```python
from build123d import *

# Parameters (mm, degrees)
SKETCH_1_R               = 1.5
SKETCH_1_R_2             = 9
SKETCH_1_R_3             = 2
EXTRUDE_1_DEPTH          = 2
CUT_EXTRUDE_1_DEPTH      = 100.85333965
CUT_EXTRUDE_1_DEPTH_BACK = 100.85333965
SKETCH_2_R               = 1.5
CUT_EXTRUDE_2_DEPTH      = 100.85333965
CUT_EXTRUDE_2_DEPTH_BACK = 100.85333965


with BuildPart() as part:
    # 草图1 → 凸台-拉伸1 (new body)
    with BuildSketch(Plane(origin=(0, 0, 0), x_dir=(1, 0, 0), z_dir=(0, 1, 0))):
        with BuildLine():
            Line((0, 47), (75.321800738, 47))
            ThreePointArc((75.321800738, 47), (76.607375957, 46.532088886), (77.291416244, 45.347296355))
            Line((77.291416244, 45.347296355), (88.047362067, -15.652703645))
            ThreePointArc((88.047362067, -15.652703645), (87.609835447, -17.285575219), (86.077746561, -18))
            Line((86.077746561, -18), (64.077746561, -18))
            ThreePointArc((64.077746561, -18), (48.289235397, -21.406433974), (35.309770387, -31.019673035))
            ThreePointArc((35.309770387, -31.019673035), (-42.818948099, -19.378794691), (0, 47))
        make_face()
        with Locations(Location((-16.264045876, 39.264880132, 0), (0, 0, 270))):
            Circle(SKETCH_1_R, mode=Mode.SUBTRACT)
        with Locations(Location((16.264045876, 39.264880132, 0), (0, 0, 270))):
            Circle(SKETCH_1_R, mode=Mode.SUBTRACT)
        with Locations(Location((39.264880132, -16.264045876, 0), (0, 0, 270))):
            Circle(SKETCH_1_R, mode=Mode.SUBTRACT)
        with Locations(Location((16.264045876, -39.264880132, 0), (0, 0, 270))):
            Circle(SKETCH_1_R, mode=Mode.SUBTRACT)
        with Locations(Location((-16.264045876, -39.264880132, 0), (0, 0, 270))):
            Circle(SKETCH_1_R, mode=Mode.SUBTRACT)
        with Locations(Location((-39.264880132, -16.264045876, 0), (0, 0, 270))):
            Circle(SKETCH_1_R, mode=Mode.SUBTRACT)
        with Locations(Location((-39.264880132, 16.264045876, 0), (0, 0, 270))):
            Circle(SKETCH_1_R, mode=Mode.SUBTRACT)
        with Locations(Location((0, 0, 0), (0, 0, 270))):
            Circle(SKETCH_1_R_2, mode=Mode.SUBTRACT)
        with Locations(Location((-6.783865663, 11.75, 0), (0, 0, 270))):
            Circle(SKETCH_1_R, mode=Mode.SUBTRACT)
        with Locations(Location((6.783865663, 11.75, 0), (0, 0, 270))):
            Circle(SKETCH_1_R, mode=Mode.SUBTRACT)
        with Locations(Location((13.567731326, 0, 0), (0, 0, 270))):
            Circle(SKETCH_1_R, mode=Mode.SUBTRACT)
        with Locations(Location((6.783865663, -11.75, 0), (0, 0, 270))):
            Circle(SKETCH_1_R, mode=Mode.SUBTRACT)
        with Locations(Location((-6.783865663, -11.75, 0), (0, 0, 270))):
            Circle(SKETCH_1_R, mode=Mode.SUBTRACT)
        with Locations(Location((-13.567731326, 0, 0), (0, 0, 270))):
            Circle(SKETCH_1_R, mode=Mode.SUBTRACT)
        with Locations(Location((0, 13.856406461, 0), (0, 0, 270))):
            Circle(SKETCH_1_R_3, mode=Mode.SUBTRACT)
        with Locations(Location((-12, -6.92820323, 0), (0, 0, 270))):
            Circle(SKETCH_1_R_3, mode=Mode.SUBTRACT)
        with Locations(Location((12, -6.92820323, 0), (0, 0, 270))):
            Circle(SKETCH_1_R_3, mode=Mode.SUBTRACT)
    extrude(amount=EXTRUDE_1_DEPTH)

    # 草图2 → 切除-拉伸1 (cut, two sides: drawn at the far end of the back side and taken through both)
    with BuildSketch(Plane(origin=(0, 2, 0), x_dir=(1, 0, 0), z_dir=(0, 1, 0)).offset(-CUT_EXTRUDE_1_DEPTH_BACK)):
        with Locations(Location((74.70156336, 37, 0), (0, 0, 270))):
            Circle(SKETCH_2_R)
        with Locations(Location((78.668920425, 14.5, 0), (0, 0, 270))):
            Circle(SKETCH_2_R)
        with Locations(Location((82.636277491, -8, 0), (0, 0, 270))):
            Circle(SKETCH_2_R)
        with Locations(Location((38.146205332, 37, 0), (0, 0, 270))):
            Circle(SKETCH_2_R)
        with Locations(Location((46.080919464, -8, 0), (0, 0, 270))):
            Circle(SKETCH_2_R)
        with Locations(Location((42.113562398, 14.5, 0), (0, 0, 270))):
            Circle(SKETCH_2_R)
        with BuildLine():
            Line((64.216309798, 27.359582102), (68.383866062, 3.72419603))
            ThreePointArc((68.383866062, 3.72419603), (63.51690861, -3.226539554), (56.566173025, 1.640417898))
            Line((56.566173025, 1.640417898), (52.398616761, 25.27580397))
            ThreePointArc((52.398616761, 25.27580397), (57.265574214, 32.226539554), (64.216309798, 27.359582102))
        make_face()
    extrude(amount=CUT_EXTRUDE_1_DEPTH + CUT_EXTRUDE_1_DEPTH_BACK, mode=Mode.SUBTRACT)

    # 草图3 → 切除-拉伸2 (cut, two sides: drawn at the far end of the back side and taken through both)
    with BuildSketch(Plane.XZ.offset(-CUT_EXTRUDE_2_DEPTH_BACK)):
        with BuildLine():
            ThreePointArc((7.550595775, -18.519948797), (12.17522858, -15.867066806), (15.934658856, -12.086630926))
            ThreePointArc((15.934658856, -12.086630926), (18.33030278, -10.583005244), (21.121590627, -11.039855496))
            Line((21.121590627, -11.039855496), (29.830018752, -16.067668818))
            ThreePointArc((29.830018752, -16.067668818), (31.73567133, -18.668128181), (31.104138605, -21.829625778))
            ThreePointArc((31.104138605, -21.829625778), (23.132934302, -30.147426931), (13.035455865, -35.694213682))
            ThreePointArc((13.035455865, -35.694213682), (9.818230989, -35.485971662), (7.799599311, -32.972204212))
            Line((7.799599311, -32.972204212), (5.197011625, -23.259214737))
            ThreePointArc((5.197011625, -23.259214737), (5.478166623, -20.44479617), (7.550595775, -18.519948797))
        make_face()
        with BuildLine():
            ThreePointArc((-12.263448247, -15.798982153), (-7.653668647, -18.47759065), (-2.5, -19.843134833))
            ThreePointArc((-2.5, -19.843134833), (0, -21.166010489), (1, -23.8117618))
            Line((1, -23.8117618), (1, -33.867388444))
            ThreePointArc((1, -33.867388444), (-0.29923758, -36.817961668), (-3.352941176, -37.851787084))
            ThreePointArc((-3.352941176, -37.851787084), (-14.54197043, -35.107422235), (-24.394367884, -29.13614277))
            ThreePointArc((-24.394367884, -29.13614277), (-25.822637443, -26.245823287), (-24.654966811, -23.240753248))
            Line((-24.654966811, -23.240753248), (-17.544565022, -16.130351459))
            ThreePointArc((-17.544565022, -16.130351459), (-14.966629547, -14.966629547), (-12.263448247, -15.798982153))
        make_face()
        with BuildLine():
            ThreePointArc((-19.814044022, 2.720966644), (-19.828897227, -2.610523844), (-18.434658856, -7.756503907))
            ThreePointArc((-18.434658856, -7.756503907), (-18.33030278, -10.583005244), (-20.121590627, -12.771906304))
            Line((-20.121590627, -12.771906304), (-28.830018752, -17.799719626))
            ThreePointArc((-28.830018752, -17.799719626), (-32.03490891, -18.149833488), (-34.457079782, -16.022161306))
            ThreePointArc((-34.457079782, -16.022161306), (-37.674904732, -4.959995304), (-37.429823749, 6.558070912))
            ThreePointArc((-37.429823749, 6.558070912), (-35.640868431, 9.240148374), (-32.454566122, 9.731450963))
            Line((-32.454566122, 9.731450963), (-22.741576647, 7.128863277))
            ThreePointArc((-22.741576647, 7.128863277), (-20.44479617, 5.478166623), (-19.814044022, 2.720966644))
        make_face()
        with BuildLine():
            ThreePointArc((-7.550595775, 18.519948797), (-12.17522858, 15.867066806), (-15.934658856, 12.086630926))
            ThreePointArc((-15.934658856, 12.086630926), (-18.33030278, 10.583005244), (-21.121590627, 11.039855496))
            Line((-21.121590627, 11.039855496), (-29.830018752, 16.067668818))
            ThreePointArc((-29.830018752, 16.067668818), (-31.73567133, 18.668128181), (-31.104138605, 21.829625778))
            ThreePointArc((-31.104138605, 21.829625778), (-23.132934302, 30.147426931), (-13.035455865, 35.694213682))
            ThreePointArc((-13.035455865, 35.694213682), (-9.818230989, 35.485971662), (-7.799599311, 32.972204212))
            Line((-7.799599311, 32.972204212), (-5.197011625, 23.259214737))
            ThreePointArc((-5.197011625, 23.259214737), (-5.478166623, 20.44479617), (-7.550595775, 18.519948797))
        make_face()
        with BuildLine():
            ThreePointArc((12.263448247, 15.798982153), (7.653668647, 18.47759065), (2.5, 19.843134833))
            ThreePointArc((2.5, 19.843134833), (0, 21.166010489), (-1, 23.8117618))
            Line((-1, 23.8117618), (-1, 33.867388444))
            ThreePointArc((-1, 33.867388444), (0.29923758, 36.817961668), (3.352941176, 37.851787084))
            ThreePointArc((3.352941176, 37.851787084), (14.54197043, 35.107422235), (24.394367884, 29.13614277))
            ThreePointArc((24.394367884, 29.13614277), (25.822637443, 26.245823287), (24.654966811, 23.240753248))
            Line((24.654966811, 23.240753248), (17.544565022, 16.130351459))
            ThreePointArc((17.544565022, 16.130351459), (14.966629547, 14.966629547), (12.263448247, 15.798982153))
        make_face()
        with BuildLine():
            ThreePointArc((19.814044022, -2.720966644), (19.828897227, 2.610523844), (18.434658856, 7.756503907))
            ThreePointArc((18.434658856, 7.756503907), (18.33030278, 10.583005244), (20.121590627, 12.771906304))
            Line((20.121590627, 12.771906304), (28.830018752, 17.799719626))
            ThreePointArc((28.830018752, 17.799719626), (32.03490891, 18.149833488), (34.457079782, 16.022161306))
            ThreePointArc((34.457079782, 16.022161306), (37.674904732, 4.959995304), (37.429823749, -6.558070912))
            ThreePointArc((37.429823749, -6.558070912), (35.640868431, -9.240148374), (32.454566122, -9.731450963))
            Line((32.454566122, -9.731450963), (22.741576647, -7.128863277))
            ThreePointArc((22.741576647, -7.128863277), (20.44479617, -5.478166623), (19.814044022, -2.720966644))
        make_face()
    extrude(amount=CUT_EXTRUDE_2_DEPTH + CUT_EXTRUDE_2_DEPTH_BACK, mode=Mode.SUBTRACT)


solid = part.part
```
Input: part model. Units: mm. Frame: model coordinates. Round coordinates to 2 decimals unless told otherwise and drop trailing zeros. Loops run counter-clockwise (first coordinate to the right, second up) from the corner with the lowest first, then second, coordinate; pieces in that order, holes last. Notation, with made-up numbers: M 39,58.25 L 61,58.25 A38 ccw 61,96.25 Z; hole C 3,-38.5 d3. An arc over 180 degrees is marked long. Answer in a Markdown table with one row per item. Add a question column.
1. Mould query, pull axis X, two halves, no side actions, for faces 1 (the face through (36, 0, -11)), 2 (the face through (12, 1, -16)). Classes: released by +X, released by -X, zero draft, split by the parting line, or undercut.
2. Ray query, probe 1 along Z at (x, y) = (18, 0.6); probe 2 along Z at (x, y) = (-27, 0.35); probe 3 along X at (y, z) = (1.85, -22.5). Return the intervals inside material, ascending.
3. Contact query for a flat-ended pin moving along its axis: pin 1 (0.6 mm diameter, centred on y = 1.5, z = -27, fed in from -X). Output: stop coordinate, or through.
4. Section A-A (y = 0.7). Give the number of separate pieces and of enclosed holes in the cut face, and give its area (3 significant figures).
5. Section B-B (x = 50.5). Output: boundary loops of the cut face in (y, z), and give its area (3 significant figures).
Values follow:
| question | item | result |
|---|---|---|
| 1 | face 1 | zero draft |
| 1 | face 2 | undercut |
| 2 | probe 1 | -47 to -33.47, -10.66 to 16.59, 33.47 to 43.42 |
| 2 | probe 2 | -38.47 to -16.74, 8.27 to 14.43, 26.74 to 38.47 |
| 2 | probe 3 | -41.26 to -23.91, 0.78 to 5.07, 30.62 to 52.89, 65.07 to 81.32 |
| 3 | pin 1 | x = -38.68 |
| 4 | separate pieces | 1 |
| 4 | enclosed holes | 30 |
| 4 | area | 6,390 mm^2 |
| 5 | outline | M 0,-47 L 2,-47 L 2,20.49 L 0,20.49 Z |
| 5 | area | 135 mm^2 |
